Verification items for the finished model (mm, model axes). A direction names the side the tool comes from. Coordinates: 2 decimals unless noted, no trailing zeros. Order: outer loops, then holes, each group sorted by start corner. A loop starts at its lowest first (then second) coordinate and runs counter-clockwise, first axis right, second up.
Q1. Set-up check for faces 1 (the flat face through (0, 0, 2.5)), 2 (the flat face through (0, 0, 0)): record each of +Z, -Z, +X, -X, +Y, -Y from which the full face is reachable in a straight line by a thin tool's end or side.
Q2. Draft check along X on faces 3 (the cylindrical face through (-21.625, -16.581, 6.916)), 4 (the flat face through (6, -26, 13)), 5 (the cylindrical face through (14.246, 22.345, 7.33)), 6 (the flat face through (10, -21, 1)). Enter one of: pulls with the +X half, pulls with the -X half, needs draft (parallel to the pull), parting line crosses it, or undercut.
Q3. Depth check by flat-ended pin: P1, Ø15.5, axis at x = -5, y = 4.5, coming from the +Z side; P2, Ø2, axis at y = 20, z = 6, coming from the -X side; P3, Ø4, axis at y = 4, z = 7.5, coming from the +X side. Enter the tip coordinate at first touch or a pass-through.
Q4. Cross-section at C-C, the plane z = 5.25. Record the boundary of the cut face in (x, y).
Q5. Thickness scan on line 1 (Y direction, x = 0, z = 4.5); line 2 (Z direction, x = -10, y = -8); line 3 (X direction, y = 6, z = 9). Record the ranges inside material, lowest first.
from build123d import *

# Parameters (mm, degrees)
F0_R     = 27.25
F1_DEPTH = 13
F2_R     = 26.5
F3_DEPTH = 12
F4_R     = 23
F5_DEPTH = 1.5
F6_R     = 1.49999
F7_R     = 1
F8_R     = 0.5


# Not quite as in the source:
# - a fillet or chamfer is up to 0.001 mm smaller than in the source, because OpenCascade refuses the exact size


with BuildPart() as f1:
    # F0 (on Top) → F1 (new body)
    with BuildSketch(Plane.XY):
        Circle(F0_R)
    extrude(amount=F1_DEPTH)

    # F2 (on face) → F3 (cut)
    with BuildSketch(Plane.XY.offset(13)):
        Circle(F2_R)
    extrude(amount=-F3_DEPTH, mode=Mode.SUBTRACT)

    # F4 (on face) → F5 (join)
    with BuildSketch(Plane.XY.offset(1)):
        Circle(F4_R)
    extrude(amount=F5_DEPTH)

    # F6 (radius 1.5 in the source; OpenCascade refuses exactly that, so slightly less here)
    f6_edges = [f1.edges().sort_by_distance(p)[0] for p in [
        (-23, 0, 2.5),
    ]]
    fillet(f6_edges, radius=F6_R)

    # F7
    f7_edges = [f1.edges().sort_by_distance(p)[0] for p in [
        (-27.25, 0, 0),
    ]]
    fillet(f7_edges, radius=F7_R)

    # F8
    f8_edges = [f1.edges().sort_by_distance(p)[0] for p in [
        (-26.5, 0, 1),
    ]]
    fillet(f8_edges, radius=F8_R)


solid = f1.part
Check values:
1. face 1: +Z
1. face 2: -Z, +X, -X, +Y, -Y
2. face 3: parting line crosses it
2. face 4: needs draft
2. face 5: undercut
2. face 6: undercut
3. P1: stops at z = 2.5
3. P2: stops at x = -19.53
3. P3: stops at x = 27.18
4. outline: circle Ø54.5 at (0, 0); hole circle Ø53 at (0, 0)
5. line 1: y = -27.25 to -26.5, 26.5 to 27.25
5. line 2: z = 0 to 2.5
5. line 3: x = -26.58 to -25.81, 25.81 to 26.58
